Verification items for the finished model (mm, model axes). A direction names the side the tool comes from. Round coordinates to 2 decimals unless told otherwise and drop trailing zeros. Write each loop counter-clockwise with the first axis right and the second up, starting at its lowest first coordinate (ties: lowest second). Pieces come first, ordered by that corner, then holes. Notation, with made-up numbers: M 81,-22 L 92,-22 A25 cw 92,14 Z; hole C 40,13 d4. An arc over 180 degrees is marked long. Answer in a Markdown table with one row per item. Add a question column.
1. Set-up check for faces 4 (the cylindrical face through (-27.15, 30.6, 1.48)), 5 (the flat face through (37.5, -23, 3)), 6 (the flat face through (1, 36, 3)), 7 (the flat face through (-41, -10, 3)), 8 (the flat face through (43.5, 0, 3)): record each of +Z, -Z, +X, -X, +Y, -Y from which the full face is reachable in a straight line by a thin tool's end or side.
2. Sectioned sample at C-C on y = -32.5. Record the cut outline in (x, z).
3. Sectioned sample at B-B on z = 1.2. Count the separate pieces of the cut face and the enclosed holes in it, plus the area to 3 significant figures.
4. Draft check along Y on faces 1 (the flat face through (-29, 31, 3)), 2 (the flat face through (-1, -36, 3)), 3 (the flat face through (-1, 1, 0)). Enter one of: pulls with the +Y half, pulls with the -Y half, needs draft (parallel to the pull), parting line crosses it, or undercut.
5. Go/stop test with flat-tipped pins: pin 1 Ø4 at (x, y) = (-28, -20) entering from -Z; pin 2 Ø2 at (x, y) = (-28, 20) entering from -Z; pin 3 Ø3 at (y, z) = (25, 3) entering from -X. Record where each tip stops, or that it passes through.
6. Material ranges on probe 1 along X at (y, z) = (-32.5, 2); probe 2 along X at (y, z) = (-20, 4.75); probe 3 along Z at (x, y) = (-29.5, 31), recorded low to high.
7. Sectioned sample at A-A on y = -20. Record the cut outline in (x, z), plus the area to 3 significant figures.
```python
from build123d import *

# Parameters (mm, degrees)
F0_W     = 6
F0_H     = 20
F1_DEPTH = 6
F2_R     = 2.25
F2_R_2   = 1.25
F2_R_3   = 1.143
F3_DEPTH = 3
F4_DEPTH = 6


with BuildPart() as f1:
    # F0 (on Top) → F1 (new body)
    with BuildSketch(Plane.XY):
        Polygon((-37.5, -36), (37.5, -36), (37.5, -10), (37.5, 10), (37.5, 36), (-37.5, 36), (-37.5, 10), (-37.5, -10), align=None)
        with Locations((40.5, 0)):
            Rectangle(F0_W, F0_H)
        with Locations((-40.5, 0)):
            Rectangle(F0_W, F0_H)
    extrude(amount=F1_DEPTH)

    # F2 (on face) → F3 (cut)
    with BuildSketch(Plane(origin=(0, 0, 0), x_dir=(1, 0, 0), z_dir=(0, 0, -1))):
        with Locations((-28, -20)):
            Circle(F2_R)
        with Locations((-28, -20)):
            Circle(F2_R_2, mode=Mode.SUBTRACT)
        with Locations((28, -20)):
            Circle(F2_R)
        with Locations((28, -20)):
            Circle(F2_R_2, mode=Mode.SUBTRACT)
        with Locations((-28, 20)):
            Circle(F2_R)
        with Locations((-28, 20)):
            Circle(F2_R_2, mode=Mode.SUBTRACT)
        with Locations((28, 20)):
            Circle(F2_R)
        with Locations((28, 20)):
            Circle(F2_R_2, mode=Mode.SUBTRACT)
        with Locations((-28.357, -32.5)):
            Circle(F2_R)
        with Locations((-28.357, -32.5)):
            Circle(F2_R_3, mode=Mode.SUBTRACT)
        with Locations((28.357, -32.5)):
            Circle(F2_R)
        with Locations((28.357, -32.5)):
            Circle(F2_R_3, mode=Mode.SUBTRACT)
        with Locations((-28.357, 32.5)):
            Circle(F2_R)
        with Locations((-28.357, 32.5)):
            Circle(F2_R_3, mode=Mode.SUBTRACT)
        with Locations((28.357, 32.5)):
            Circle(F2_R)
        with Locations((28.357, 32.5)):
            Circle(F2_R_3, mode=Mode.SUBTRACT)
    extrude(amount=-F3_DEPTH, mode=Mode.SUBTRACT)

    # F2 (on face) → F4 (cut, through all)
    with BuildSketch(Plane(origin=(0, 0, 0), x_dir=(1, 0, 0), z_dir=(0, 0, -1))):
        with Locations((-28, 20)):
            Circle(F2_R_2)
        with Locations((-28, -20)):
            Circle(F2_R_2)
        with Locations((28, -20)):
            Circle(F2_R_2)
        with Locations((28, 20)):
            Circle(F2_R_2)
        with Locations((-28.357, -32.5)):
            Circle(F2_R_3)
        with Locations((28.357, -32.5)):
            Circle(F2_R_3)
        with Locations((28.357, 32.5)):
            Circle(F2_R_3)
        with Locations((-28.357, 32.5)):
            Circle(F2_R_3)
    extrude(amount=-F4_DEPTH, mode=Mode.SUBTRACT)


solid = f1.part
```
Geometry check:
| question | item | result |
|---|---|---|
| 1 | face 4 | -Z |
| 1 | face 5 | +Z, -Z, +X, -Y |
| 1 | face 6 | +Z, -Z, +X, -X, +Y |
| 1 | face 7 | +Z, -Z, -X, -Y |
| 1 | face 8 | +Z, -Z, +X, +Y, -Y |
| 2 | outline | M -37.5,0 L -30.61,0 L -30.61,3 L -29.5,3 L -29.5,6 L -37.5,6 Z; M -27.21,3 L -26.11,3 L -26.11,0 L 26.11,0 L 26.11,3 L 27.21,3 L 27.21,6 L -27.21,6 Z; M 29.5,3 L 30.61,3 L 30.61,0 L 37.5,0 L 37.5,6 L 29.5,6 Z |
| 3 | separate pieces | 1 |
| 3 | enclosed holes | 8 |
| 3 | area | 5,510 mm2 |
| 4 | face 1 | undercut |
| 4 | face 2 | pulls with the -Y half |
| 4 | face 3 | needs draft |
| 5 | pin 1 | stops at z = 3 |
| 5 | pin 2 | passes through |
| 5 | pin 3 | stops at x = -37.5 |
| 6 | probe 1 | x = -37.5 to -30.61, -26.11 to 26.11, 30.61 to 37.5 |
| 6 | probe 2 | x = -37.5 to -29.25, -26.75 to 26.75, 29.25 to 37.5 |
| 6 | probe 3 | z = 3 to 6 |
| 7 | outline | M -37.5,0 L -30.25,0 L -30.25,3 L -29.25,3 L -29.25,6 L -37.5,6 Z; M -26.75,3 L -25.75,3 L -25.75,0 L 25.75,0 L 25.75,3 L 26.75,3 L 26.75,6 L -26.75,6 Z; M 29.25,3 L 30.25,3 L 30.25,0 L 37.5,0 L 37.5,6 L 29.25,6 Z |
| 7 | area | 408 mm2 |
